from build123d import *

# Parameters (mm, degrees)
SKETCH_R     = 3.05
PAD_DEPTH    = 3.6
SKETCH001_R  = 5
PAD001_DEPTH = 6
SKETCH002_R  = 3.2
POCKET_DEPTH = 4
CHAMFER_SIZE = 0.4


with BuildPart() as part:
    # Sketch → Pad (new body)
    with BuildSketch(Plane.XY):
        Circle(SKETCH_R)
    extrude(amount=PAD_DEPTH)

    # Sketch001 → Pad001 (new body)
    with BuildSketch(Plane.XY.offset(3.6)):
        Circle(SKETCH001_R)
    extrude(amount=PAD001_DEPTH)

    # Sketch002 → Pocket (cut)
    with BuildSketch(Plane.XY.offset(9.6)):
        Circle(SKETCH002_R)
    extrude(amount=-POCKET_DEPTH, mode=Mode.SUBTRACT)

    # Chamfer
    chamfer_edges = [part.edges().sort_by_distance(p)[0] for p in [
        (-3.2, 0, 9.6),
    ]]
    chamfer(chamfer_edges, length=CHAMFER_SIZE)


solid = part.part
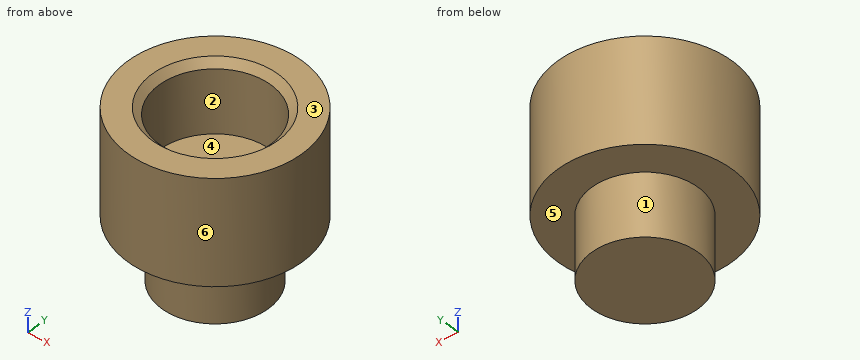
Geometry: final body of the model. Coordinates: model frame, mm. Face numbers are marked on the shaded views. A direction names the side the tool comes from. Coordinates: 2 decimals unless noted, no trailing zeros. Order: outer loops, then holes, each group sorted by start corner. A loop starts at its lowest first (then second) coordinate and runs counter-clockwise, first axis right, second up. Notation, with made-up numbers: (59, -28.75) - (71, -28.75) arc R27 cw to (71, 8.25) - close; hole circle Ø4 at (3, 35). An arc over 180 degrees is marked (long way). Use one line per item in the form item = value.
1) Section A-A (y = 0). Return loops of the section in (x, z), then the cut area to 3 significant figures.
Solutions:
outline = (-5, 3.6) - (-3.05, 3.6) - (-3.05, 0) - (3.05, 0) - (3.05, 3.6) - (5, 3.6) - (5, 9.6) - (3.6, 9.6) - (3.2, 9.2) - (3.2, 5.6) - (-3.2, 5.6) - (-3.2, 9.2) - (-3.6, 9.6) - (-5, 9.6) - close
area = 56.2 mm^2
2) Set-up query: the marked faces 4, 5 and 6. Return all of +Z, -Z, +X, -X, +Y, -Y with unobstructed straight access to the full face (end or side cutting, diameter ignored); none if empty.
Solutions:
face_4 = +Z
face_5 = -Z
face_6 = +Z, -Z
3) Section C-C (z = 6.25). Return loops of the section in (x, y).
Solutions:
outline = circle Ø10 at (0, 0); hole circle Ø6.4 at (0, 0)
4) Pin query (flat end, axial travel): pin 1 (6 mm diameter, centred on x = -1.5, y = 0.5, fed in from +Z); pin 2 (1.5 mm diameter, centred on y = -1.5, z = 8, fed in from -X); pin 3 (2 mm diameter, centred on x = -3, z = 3.5, fed in from -Y); pin 4 (1 mm diameter, centred on x = 1, z = 5, fed in from -Y). Return the tip coordinate at first contact, or that it passes through.
Solutions:
pin_1 = 9.6
pin_2 = -4.94
pin_3 = -4.58
pin_4 = -4.97
5) Mould query, pull axis Y, two halves, no side actions, for the marked faces 1, 2 and 3. Classes: +Y half, -Y half, draft (parallel to the pull), parting line (faces both ways), or undercut.
Solutions:
face_1 = parting line
face_2 = undercut
face_3 = draft
6) Section D-D (z = 2.5). Return loops of the section in (x, y), then the cut area to 3 significant figures.
Solutions:
outline = circle Ø6.1 at (0, 0)
area = 29.2 mm^2
7) Ray query, L1, parallel to Y at x = 0, z = 7.6; L2, parallel to Z at x = -0.25, y = -4; L3, parallel to Z at x = -0.75, y = 1. Return the intervals inside material, ascending.
Solutions:
L1 = -5 to -3.2, 3.2 to 5
L2 = 3.6 to 9.6
L3 = 0 to 5.6
